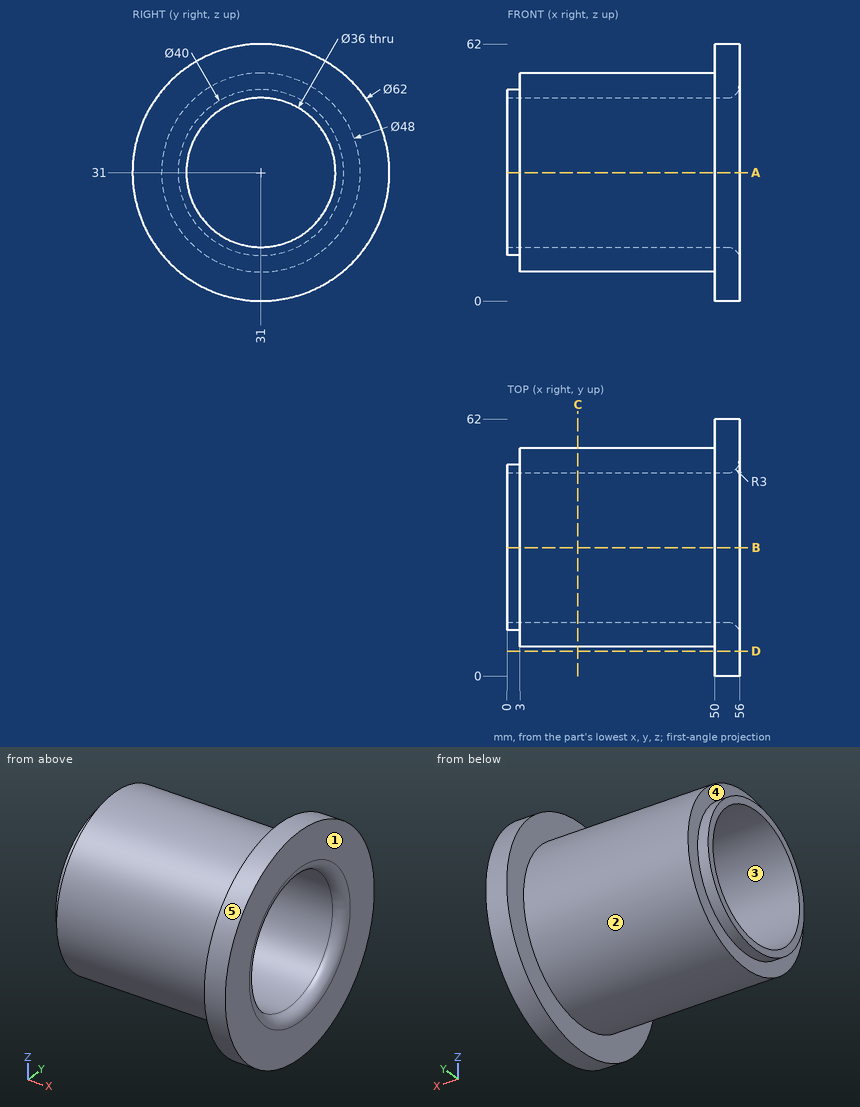
Verification items for this drawing (mm, ordinates from the low corner). A direction names the side the tool comes from. Coordinates: 2 decimals unless noted, no trailing zeros. Order: outer loops, then holes, each group sorted by start corner. A loop starts at its lowest first (then second) coordinate and runs counter-clockwise, first axis right, second up. Notation, with made-up numbers: (19.25, -23.5) - (76.25, -23.5) arc R28 cw to (76.25, 4.5) - close; hole circle Ø1 at (11, -22.5). An arc over 180 degrees is marked (long way). Answer as a JSON object with one key per item and string values. Group by question number.
Item 1: Tool access check on the marked faces 4 and 5. Record the directions out of +Z, -Z, +X, -X, +Y, -Y that give a thin tool (end or side, any length) a straight path to the whole face; none if there is none.
Item 2: Sectioned sample at A-A, the plane z = 31. Record the cut outline in (x, y).
Item 3: Scan lines: probe 1 along Y at (x, z) = (39, 31); probe 2 along Z at (x, y) = (10, 36); probe 3 along Y at (x, z) = (31, 28). Record each from-to range of solid material in increasing order.
Item 4: Depth check by flat-ended pin: pin 1 Ø6 at (x, y) = (27.5, 54) entering from -Z; pin 2 Ø2 at (y, z) = (41, 51) entering from -X; pin 3 Ø1.5 at (x, y) = (12, 9.5) entering from -Z. Enter the tip coordinate at first touch or a pass-through.
Item 5: Sectioned sample at D-D, the plane y = 6. Record the cut outline in (x, z).
Item 6: Sectioned sample at C-C, the plane x = 17. Record the cut outline in (y, z).
Item 7: Draft check along Y on the marked faces 1, 2 and 3. Enter one of: +Y half, -Y half, draft (parallel to the pull), parting line (faces both ways), or undercut.
Resolved:
{
 "1": {"face 4": "-X", "face 5": "+X, -X"},
 "2": {"outline": "(0, 11) - (3, 11) - (3, 7) - (50, 7) - (50, 0) - (56, 0) - (56, 10) arc R3 ccw to (53, 13) - (0, 13) - close; (0, 49) - (53, 49) arc R3 ccw to (56, 52) - (56, 62) - (50, 62) - (50, 55) - (3, 55) - (3, 51) - (0, 51) - close"},
 "3": {"probe 1": "7 to 13, 49 to 55", "probe 2": "7.53 to 13.71, 48.29 to 54.47", "probe 3": "7.19 to 13.25, 48.75 to 54.81"},
 "4": {"pin 1": "z = 17.73", "pin 2": "x = 3", "pin 3": "z = 18.94"},
 "5": {"outline": "(50, 12.67) - (56, 12.67) - (56, 49.33) - (50, 49.33) - close"},
 "6": {"outline": "circle Ø48 at (31, 31); hole circle Ø36 at (31, 31)"},
 "7": {"face 1": "draft", "face 2": "parting line", "face 3": "undercut"}
}
